from build123d import *

# Parameters (mm, degrees)
F0_W     = 19.05
F0_H     = 152.4
F0_W_2   = 203.2
F0_H_2   = 203.2
F0_R     = 13.335
F1_DEPTH = 19.05


with BuildPart() as f1:
    # F0 (on Top) → F1 (new body)
    with BuildSketch(Plane.XY):
        Polygon((-305.997565, 1118.248048), (-305.997565, -100.951952), (-102.797565, -100.951952), (100.402435, -100.951952), (303.602435, -100.951952), (303.602435, 1118.248048), (57.15, 1118.248048), (57.15, 686.448048), (-57.15, 686.448048), (-57.15, 1118.248048), align=None)
        with Locations((-269.875, 329.650346)):
            Rectangle(F0_W, F0_H, mode=Mode.SUBTRACT)
        with Locations((270.383059, 329.650346)):
            Rectangle(F0_W, F0_H, mode=Mode.SUBTRACT)
        Polygon((76.2, 507.704346), (76.2, 498.179346), (76.2, 488.654346), (-76.2, 488.654346), (-76.2, 498.179346), (-76.2, 507.704346), align=None, mode=Mode.SUBTRACT)
        with Locations((-1.197565, -202.551952)):
            Rectangle(F0_W_2, F0_H_2)
        with Locations((-1.197565, -202.551952)):
            Circle(F0_R, mode=Mode.SUBTRACT)
    extrude(amount=F1_DEPTH)


solid = f1.part
CAD build for the part. Positions are in the model's coordinates, mm. Round coordinates to 2 decimals unless told otherwise and drop trailing zeros. Write each loop counter-clockwise with the first axis right and the second up, starting at its lowest first coordinate (ties: lowest second). Pieces come first, ordered by that corner, then holes.
(1) Slice it at C-C, the plane x = 181. Write the cut outline in (y, z).
(2) Mould opens along Y. For faces 1 (the face through (-4.09, -215.57, 9.39)), 2 (the face through (-5, 417, 0)) say: pulls with the +Y half, pulls with the -Y half, needs draft (parallel to the pull), parting line crosses it, or undercut.
(3) Drop a flat-ended pin along its axis: P1, Ø5.5, axis at x = -271.5, z = 11, coming from the -Y side. Give the stop position or say it passes through.
(4) Probe line 1 along Y through (x, z) = (68, 3.5); line 2 along X through (y, z) = (335, 11.5); line 3 along X through (y, z) = (1042, 16.75). List the from-to ranges inside material, lowest first.
(5) Slice it at A-A, the plane y = 350. Write the cut outline in (x, z), and give its area (3 significant figures).
(6) Slice it at B-B, the plane z = 16. Write the cut outline in (x, y) (3 decimals), and give its area (3 significant figures).
From the geometry:
1. outline: (-100.95, 0) - (1118.25, 0) - (1118.25, 19.05) - (-100.95, 19.05) - close
2. face 1: undercut
2. face 2: needs draft
3. P1: stops at y = -100.95
4. line 1: y = -304.15 to 488.65, 507.7 to 1118.25
4. line 2: x = -306 to -279.4, -260.35 to 260.86, 279.91 to 303.6
4. line 3: x = -306 to -57.15, 57.15 to 303.6
5. outline: (-306, 0) - (-279.4, 0) - (-279.4, 19.05) - (-306, 19.05) - close; (-260.35, 0) - (260.86, 0) - (260.86, 19.05) - (-260.35, 19.05) - close; (279.91, 0) - (303.6, 0) - (303.6, 19.05) - (279.91, 19.05) - close
5. area: 10,900 mm2
6. outline: (-305.998, -100.952) - (-102.798, -100.952) - (-102.798, -304.152) - (100.402, -304.152) - (100.402, -100.952) - (303.602, -100.952) - (303.602, 1118.248) - (57.15, 1118.248) - (57.15, 686.448) - (-57.15, 686.448) - (-57.15, 1118.248) - (-305.998, 1118.248) - close; hole (-279.4, 253.45) - (-260.35, 253.45) - (-260.35, 405.85) - (-279.4, 405.85) - close; hole (-76.2, 488.654) - (76.2, 488.654) - (76.2, 507.704) - (-76.2, 507.704) - close; hole circle Ø26.67 at (-1.198, -202.552); hole (260.858, 253.45) - (279.908, 253.45) - (279.908, 405.85) - (260.858, 405.85) - close
6. area: 726,000 mm2
